Design review of the part built by this model. Coordinates are the model's own, in mm. Face numbers are marked on the shaded views. A direction names the side the tool comes from. Round coordinates to 2 decimals unless told otherwise and drop trailing zeros. Order: outer loops, then holes, each group sorted by start corner. A loop starts at its lowest first (then second) coordinate and runs counter-clockwise, first axis right, second up. Notation, with made-up numbers: M 76,54 L 95,54 A21 cw 95,59 Z; hole C 87.25,83 d10. An arc over 180 degrees is marked long. Write each question's results on one line, items separated by ' | '. Start each with the question number.
Item 1: Take a section at C-C, the plane x = -232. Write out the cut boundary in (y, z).
Item 2: Machinability: for the marked faces 4, 5 and 6, which of the approach directions +Z, -Z, +X, -X, +Y, -Y give a long, thin tool a straight path to every point of the face, cutting with its end or side? Answer none if there is none.
Item 3: Clearance check with flat-ended pins moving along their axes: pin 1 (2.5 mm diameter, centred on y = 34.5, z = 75.5, fed in from -X); pin 2 (14 mm diameter, centred on x = -222, y = 13.5, fed in from -Z); pin 3 (10.5 mm diameter, centred on y = 64.5, z = -56, fed in from -X). State where each tip first meets the part, or that it passes through.
Item 4: The part is to be moulded in two halves that separate along X. For the marked faces 1, 2 and 3, say which applies: +X half, -X half, draft (parallel to the pull), parting line (faces both ways), or undercut.
Item 5: Wall thickness on line 1 (X direction, y = 43.25, z = 0); line 2 (Z direction, x = 27, y = 64); line 3 (X direction, y = 2, z = -12): over which ranges is each line inside the solid? List them lowest first. Write a range as [from, to].
Item 6: Take a section at B-B, the plane y = 64.5. Write out the cut boundary in (x, z), plus the area to 3 significant figures.
Item 7: Take a section at A-A, the plane x = -196.5. Write out the cut boundary in (y, z).
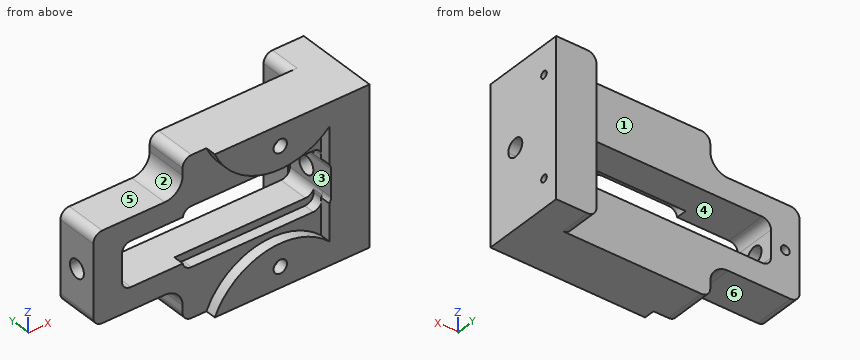
```python
from build123d import *

# Parameters (mm, degrees)
BOSS_EXTRUDE1_DEPTH = 47
BOSS_EXTRUDE2_DEPTH = 35
BOSS_EXTRUDE3_START = 12
BOSS_EXTRUDE3_DEPTH = 12
SKETCH3_R           = 4
CUT_EXTRUDE1_DEPTH  = 324.215098657
SKETCH6_R           = 7.5
CUT_EXTRUDE3_DEPTH  = 12
CUT_EXTRUDE2_DEPTH  = 12
SKETCH8_R           = 5
CUT_EXTRUDE4_DEPTH  = 14


with BuildPart() as part:
    # Sketch1 → Boss-Extrude1 (new body)
    with BuildSketch(Plane(origin=(0, 0, 0), x_dir=(1, 0, 0), z_dir=(0, 1, 0))):
        with BuildLine():
            Line((-256.288485132, 40), (-256.288485132, -40))
            ThreePointArc((-256.288485132, -40), (-253.359552944, -47.071067812), (-246.288485132, -50))
            Line((-246.288485132, -50), (-176.288485132, -50))
            ThreePointArc((-176.288485132, -50), (-162.146349509, -55.857864376), (-156.288485132, -70))
            Line((-156.288485132, -70), (-156.288485132, -78))
            ThreePointArc((-156.288485132, -78), (-153.359552944, -85.071067812), (-146.288485132, -88))
            Line((-146.288485132, -88), (43.711514868, -88))
            Line((43.711514868, -88), (43.711514868, 88))
            Line((43.711514868, 88), (-146.288485132, 88))
            ThreePointArc((-146.288485132, 88), (-153.359552944, 85.071067812), (-156.288485132, 78))
            Line((-156.288485132, 78), (-156.288485132, 70))
            ThreePointArc((-156.288485132, 70), (-162.146349509, 55.857864376), (-176.288485132, 50))
            Line((-176.288485132, 50), (-246.288485132, 50))
            ThreePointArc((-246.288485132, 50), (-253.359552944, 47.071067812), (-256.288485132, 40))
        make_face()
        with BuildLine():
            Line((-224.288485132, 15), (-224.288485132, -15))
            ThreePointArc((-224.288485132, -15), (-221.359552944, -22.071067812), (-214.288485132, -25))
            Line((-214.288485132, -25), (-9.288485132, -25))
            ThreePointArc((-9.288485132, -25), (-2.217417321, -22.071067812), (0.711514868, -15))
            Line((0.711514868, -15), (0.711514868, 15))
            ThreePointArc((0.711514868, 15), (-2.217417321, 22.071067812), (-9.288485132, 25))
            Line((-9.288485132, 25), (-214.288485132, 25))
            ThreePointArc((-214.288485132, 25), (-221.359552944, 22.071067812), (-224.288485132, 15))
        make_face(mode=Mode.SUBTRACT)
    extrude(amount=BOSS_EXTRUDE1_DEPTH)

    # Sketch2 → Boss-Extrude2 (add)
    with BuildSketch(Plane(origin=(0, 47, 0), x_dir=(1, 0, 0), z_dir=(0, 1, 0))):
        with BuildLine():
            Line((43.711514868, -88), (43.711514868, 88))
            Line((43.711514868, 88), (8.711514868, 88))
            ThreePointArc((8.711514868, 88), (1.640447056, 85.071067812), (-1.288485132, 78))
            Line((-1.288485132, 78), (-1.288485132, -78))
            ThreePointArc((-1.288485132, -78), (1.640447056, -85.071067812), (8.711514868, -88))
            Line((8.711514868, -88), (43.711514868, -88))
        make_face()
    extrude(amount=BOSS_EXTRUDE2_DEPTH)

    # Sketch7 → Boss-Extrude3 (add)
    with BuildSketch(Plane.XZ.offset(BOSS_EXTRUDE3_START)):
        with BuildLine():
            ThreePointArc((-1.288485132, -61.905249807), (-72.230589483, -41.6045326), (-129.609696252, -88))
            Line((-129.609696252, -88), (43.711514868, -88))
            Line((43.711514868, -88), (43.711514868, 88))
            Line((43.711514868, 88), (-129.609696252, 88))
            ThreePointArc((-129.609696252, 88), (-72.230589483, 41.6045326), (-1.288485132, 61.905249807))
            Line((-1.288485132, 61.905249807), (-1.288485132, 21))
            ThreePointArc((-1.288485132, 21), (0.198347848, 18.16227766), (0.711514868, 15))
            Line((0.711514868, 15), (0.711514868, -15))
            ThreePointArc((0.711514868, -15), (0.198347848, -18.16227766), (-1.288485132, -21))
            Line((-1.288485132, -21), (-1.288485132, -61.905249807))
        make_face()
    extrude(amount=-BOSS_EXTRUDE3_DEPTH)

    # Sketch3 → Cut-Extrude1 (cut, through all)
    with BuildSketch(Plane.ZY.offset(256.288485132)):
        with BuildLine():
            ThreePointArc((0, 33.5), (-10, 23.5), (0, 13.5))
            Line((0, 13.5), (0, 33.5))
        make_face()
        with BuildLine():
            Line((0, 33.5), (0, 13.5))
            ThreePointArc((0, 13.5), (7.071067812, 16.428932188), (10, 23.5))
            ThreePointArc((10, 23.5), (7.071067812, 30.571067812), (0, 33.5))
        make_face()
        with Locations((56, 64.5)):
            Circle(SKETCH3_R)
        with Locations((-56, 64.5)):
            Circle(SKETCH3_R)
    extrude(amount=-CUT_EXTRUDE1_DEPTH, mode=Mode.SUBTRACT)

    # Sketch6 → Cut-Extrude3 (cut)
    with BuildSketch(Plane.XZ):
        with Locations(Location((-56.288485132, 65, 0), (0, 0, 270))):
            Circle(SKETCH6_R)
        with Locations(Location((-56.288485132, -65, 0), (0, 0, 270))):
            Circle(SKETCH6_R)
    extrude(amount=CUT_EXTRUDE3_DEPTH, mode=Mode.SUBTRACT)

    # Sketch5 → Cut-Extrude2 (cut)
    with BuildSketch(Plane.XZ):
        with BuildLine():
            Line((0, 23), (0, -23))
            ThreePointArc((0, -23), (-2.928932188, -30.071067812), (-10, -33))
            Line((-10, -33), (-146.288485132, -33))
            ThreePointArc((-146.288485132, -33), (-153.359552944, -30.071067812), (-156.288485132, -23))
            Line((-156.288485132, -23), (-156.288485132, 23))
            ThreePointArc((-156.288485132, 23), (-153.359552944, 30.071067812), (-146.288485132, 33))
            Line((-146.288485132, 33), (-10, 33))
            ThreePointArc((-10, 33), (-2.928932188, 30.071067812), (0, 23))
        make_face()
    extrude(amount=-CUT_EXTRUDE2_DEPTH, mode=Mode.SUBTRACT)

    # Sketch8 → Cut-Extrude4 (cut)
    with BuildSketch(Plane(origin=(0, 47, 0), x_dir=(1, 0, 0), z_dir=(0, 1, 0))):
        with Locations(Location((-240.288485132, 0, 0), (0, 0, 270))):
            Circle(SKETCH8_R)
    extrude(amount=-CUT_EXTRUDE4_DEPTH, mode=Mode.SUBTRACT)


solid = part.part
```
Results list:
1) outline: M 0,-50 L 47,-50 L 47,50 L 0,50 Z; hole C 23.5,0 d20
2) face 4: +Y, -Y | face 5: +Z, -X, +Y, -Y | face 6: -Z, -X, +Y, -Y
3) pin 1: x = -156.29 | pin 2: z = -50 | pin 3: x = -1.29
4) face 1: draft | face 2: -X half | face 3: undercut
5) line 1: [-256.29, -245.29], [-235.29, -224.29], [0.71, 43.71] | line 2: [-88, -59.97], [-52.03, 52.03], [59.97, 88] | line 3: [-256.29, -224.29], [0.71, 43.71]
6) outline: M -1.29,-78 A10 ccw 8.71,-88 L 43.71,-88 L 43.71,-60 L -1.29,-60 Z; M -1.29,-52 L 43.71,-52 L 43.71,52 L -1.29,52 Z; M -1.29,60 L 43.71,60 L 43.71,88 L 8.71,88 A10 ccw -1.29,78 Z | area: 7,160 mm²
7) outline: M 0,-50 L 47,-50 L 47,-25 L 0,-25 Z; M 0,25 L 47,25 L 47,50 L 0,50 Z
